Geometry check sheet. Reference: the model listing, model coordinates, mm. A direction names the side the tool comes from. Coordinates: 2 decimals unless noted, no trailing zeros. Write each loop counter-clockwise with the first axis right and the second up, starting at its lowest first coordinate (ties: lowest second). Pieces come first, ordered by that corner, then holes. Notation, with made-up numbers: (-37, 86.5) -> (3, 86.5) arc R20 ccw to (3, 92.5) -> close; hole circle Ø9 at (65, 33.5). An arc over 180 degrees is marked (long way). One line per question, with ' | ' between items.
Solid Edge part; units mm, degrees
sketch "Sketch1" plane through (0, 0, 0) normal (0, 0, 1) x (1, 0, 0)
  line L0 (-37.5, -26) -> (37.5, -26)
  line L1 (37.5, -26) -> (37.5, 26)
  line L2 (37.5, 26) -> (-37.5, 26)
  line L3 (-37.5, 26) -> (-37.5, -26)
  circle A0 centre (-27.5, -16) radius 5
  circle A1 centre (-27.5, 16) radius 5
  circle A2 centre (27.5, 16) radius 5
  circle A3 centre (27.5, -16) radius 5
extrude "Protrusion1" add sketch "Sketch1" along normal mid plane 15
sketch "Sketch2" plane through (0, 0, 0) normal (0, -1, 0) x (1, 0, 0)
  arc A0 (-32.5, 17.5) -> (-2.5, 47.5) centre (-2.5, 17.5) cw
  line L0 (-2.5, 47.5) -> (7.5, 47.5)
  line L1 (7.5, 47.5) -> (7.5, 27.5021)
  line L2 (7.5, 27.5021) -> (-2.5, 27.5021)
  arc A1 (-12.5, 17.5) -> (-2.5, 27.5021) centre (-2.5, 17.5021) cw
  line L3 (-12.5, 17.5) -> (-12.5, 7.5)
  line L4 (-12.5, 7.5) -> (-32.5, 7.5)
  line L5 (-32.5, 7.5) -> (-32.5, 17.5)
extrude "ExtrudedProtrusion_2" add sketch "Sketch2" along normal mid plane 12
sketch "Sketch3" plane through (2.5, 0, 47.5) normal (0, 0, 1) x (0, 1, 0)
  circle A0 centre (0, -20) radius 16
  circle A1 centre (0, -20) radius 8
extrude "ExtrudedProtrusion_3" add sketch "Sketch3" against normal blind 20
(1) Draft check along Y on faces 1 (the face through (-1, 0, 7.5)), 2 (the face through (1, 26, 0)), 3 (the face through (-31.5, -13, -0.1)). Enter one of: pulls with the +Y half, pulls with the -Y half, needs draft (parallel to the pull), parting line crosses it, or undercut.
Answers below:
face 1: needs draft | face 2: pulls with the +Y half | face 3: undercut
(2) Depth check by flat-ended pin: P1, Ø10, axis at x = 19.5, z = 30, coming from the +Y side; P2, Ø4, axis at x = -15, z = 40, coming from the -Y side; P3, Ø2, axis at y = 10, z = -0.5, coming from the +X side; P4, Ø16, axis at x = 27.5, y = -16, coming from the -Z side. Enter the tip coordinate at first touch or a pass-through.
Answers below:
P1: stops at y = 16 | P2: stops at y = -6 | P3: stops at x = 37.5 | P4: stops at z = -7.5
(3) Cross-section at A-A (x = 3.5). Record the cut outline in (y, z), plus the area to 3 significant figures.
Answers below:
outline: (-26, -7.5) -> (26, -7.5) -> (26, 7.5) -> (-26, 7.5) -> close; (-6, 27.5) -> (6, 27.5) -> (6, 47.5) -> (-6, 47.5) -> close | area: 1,020 mm²
(4) Material ranges on line 1 (Y direction, x = 22.5, z = 37); line 2 (Y direction, x = -27, z = 1); line 3 (Z direction, x = 15.5, y = -5), recorded low to high.
Answers below:
line 1: y = -16 to -8, 8 to 16 | line 2: y = -26 to -20.97, -11.03 to 11.03, 20.97 to 26 | line 3: z = -7.5 to 7.5, 27.5 to 47.5
(5) Cross-section at C-C (x = -27.5). Record the cut outline in (y, z).
Answers below:
outline: (-26, -7.5) -> (-21, -7.5) -> (-21, 7.5) -> (-26, 7.5) -> close; (-11, -7.5) -> (11, -7.5) -> (11, 7.5) -> (6, 7.5) -> (6, 34.08) -> (-6, 34.08) -> (-6, 7.5) -> (-11, 7.5) -> close; (21, -7.5) -> (26, -7.5) -> (26, 7.5) -> (21, 7.5) -> close
(6) Tool access check on faces 4 (the face through (30.31, -1.73, 37.64)), 5 (the face through (37.5, 0, 0)), 6 (the face through (-12, -6, 27)), 7 (the face through (-12.5, 0, 13)). Record the directions out of +Z, -Z, +X, -X, +Y, -Y that give a thin tool (end or side, any length) a straight path to the whole face; none if there is none.
Answers below:
face 4: +Z | face 5: -Z, +X, +Y, -Y | face 6: +Z, -X, -Y | face 7: +X, +Y, -Y
(7) Cross-section at D-D (y = 17). Record the cut outline in (x, z), plus the area to 3 significant figures.
Answers below:
outline: (-37.5, -7.5) -> (-32.4, -7.5) -> (-32.4, 7.5) -> (-37.5, 7.5) -> close; (-22.6, -7.5) -> (22.6, -7.5) -> (22.6, 7.5) -> (-22.6, 7.5) -> close; (32.4, -7.5) -> (37.5, -7.5) -> (37.5, 7.5) -> (32.4, 7.5) -> close | area: 831 mm²
